Read the model definition and answer for the solid it produces. Units are mm, in the model's axes. A direction names the side the tool comes from. Coordinates: 2 decimals unless noted, no trailing zeros. Loops run counter-clockwise (first coordinate to the right, second up) from the corner with the lowest first, then second, coordinate; pieces in that order, holes last. Notation, with made-up numbers: M 48,38 L 98,38 A14 cw 98,48 Z; hole C 71.5,60 d11. An arc over 180 degrees is marked long. Put each result on its own line as item: value.
from build123d import *

# Parameters (mm, degrees)
BOSS_SWITCH_BODY_DEPTH            = 3
SKETCH1_W                         = 2.994375291
SKETCH1_H                         = 2.409101515
SKETCH1_W_2                       = 3.994375291
SKETCH1_H_2                       = 3.957767538
BOSS_FLANGE_WIDTH_DEPTH           = 5
BOSS_FLANGE_HEIGHT_REACH          = 36.354
SKETCH2_W                         = 4
SKETCH2_H                         = 3.957767538
SKETCH2_W_2                       = 8
SKETCH2_H_2                       = 1.451333978
SKETCH17_W                        = 15.1675
SKETCH17_H                        = 4
BOSS_FLANGE_SUPPORT_DEPTH         = 13.053634428
CUT_WALL_GAP_DEPTH                = 1
TAP_DRILL_FOR_M2X0_4_TAP1_D       = 1.6
M2_CLEARANCE_HOLE2_D              = 2.4
M2_CLEARANCE_HOLE2_DEPTH          = 13.462735941
CHAMFER_FLANGE_SUPPORT_3_SIZE     = 1
FILLET1_R                         = 1
FILLET2_R                         = 0.5
SKETCH28_W                        = 5.9675
SKETCH28_H                        = 12.095866891
CUT_PRINT_SUPPORT_CLEARANCE_DEPTH = 33.624103931


with BuildPart() as part:
    # Sketch-SwitchBossUp → Boss-Switch Body (new body)
    with BuildSketch(Plane.XY):
        with BuildLine():
            Line((-5.697895702, 26.949658376), (-5.524247524, 25.964850623))
            ThreePointArc((-5.524247524, 25.964850623), (-6.169751391, 25.553619307), (-6.3354071, 24.806394693))
            Line((-6.3354071, 24.806394693), (-4.07798079, 12.003893904))
            ThreePointArc((-4.07798079, 12.003893904), (-3.666749473, 11.358390037), (-2.919524859, 11.192734328))
            Line((-2.919524859, 11.192734328), (-2.816117912, 10.606284387))
            Line((-2.816117912, 10.606284387), (-1.811990528, 10.217060362))
            Line((-1.811990528, 10.217060362), (-1.182618868, 9.973100706))
            Line((-1.182618868, 9.973100706), (-1.735258621, 8.547390389))
            ThreePointArc((-1.735258621, 8.547390389), (-1.752158006, 8.457034961), (-1.735258621, 8.366679532))
            Line((-1.735258621, 8.366679532), (-1.182618868, 6.940969215))
            Line((-1.182618868, 6.940969215), (-1.811990528, 6.697009559))
            Line((-1.811990528, 6.697009559), (-0.547014535, 3.433600952))
            Line((-0.547014535, 3.433600952), (0.082357125, 3.677560608))
            Line((0.082357125, 3.677560608), (0.805200549, 1.81275569))
            Line((0.805200549, 1.81275569), (-0.12720191, 1.451333978))
            Line((-0.12720191, 1.451333978), (-0.12720191, 0))
            Line((-0.12720191, 0), (2.867173381, 0))
            Line((2.867173381, 0), (2.867173381, 2.409101515))
            Line((2.867173381, 2.409101515), (2.343664607, 2.409101515))
            Line((2.343664607, 2.409101515), (1.411262148, 2.047679803))
            Line((1.411262148, 2.047679803), (0.688418723, 3.912484721))
            Line((0.688418723, 3.912484721), (1.317790383, 4.156444377))
            Line((1.317790383, 4.156444377), (1.13533703, 4.627140933))
            Line((1.13533703, 4.627140933), (3.197473995, 5.426475025))
            Line((3.197473995, 5.426475025), (3.197473995, 6.761927069))
            Line((3.197473995, 6.761927069), (2.297289747, 7.748445958))
            Line((2.297289747, 7.748445958), (0.235267743, 6.949156428))
            Line((0.235267743, 6.949156428), (0.05281439, 7.419852984))
            Line((0.05281439, 7.419852984), (-0.57655727, 7.175893328))
            Line((-0.57655727, 7.175893328), (-1.038134762, 8.366679532))
            ThreePointArc((-1.038134762, 8.366679532), (-1.055034148, 8.457034961), (-1.038134762, 8.547390389))
            Line((-1.038134762, 8.547390389), (-0.57655727, 9.738176593))
            Line((-0.57655727, 9.738176593), (0.05281439, 9.494216937))
            Line((0.05281439, 9.494216937), (1.317790383, 12.757625544))
            Line((1.317790383, 12.757625544), (0.688418723, 13.0015852))
            Line((0.688418723, 13.0015852), (1.411262148, 14.866390118))
            Line((1.411262148, 14.866390118), (2.343664607, 14.504968406))
            Line((2.343664607, 14.504968406), (2.867173381, 14.504968406))
            Line((2.867173381, 14.504968406), (2.867173381, 18.462735944))
            Line((2.867173381, 18.462735944), (-0.111637615, 18.462735944))
            Line((-0.111637615, 18.462735944), (-1.12720191, 18.462735944))
            Line((-1.12720191, 18.462735944), (-1.12720191, 15.462735944))
            Line((-1.12720191, 15.462735944), (-0.12720191, 15.462735944))
            Line((-0.12720191, 15.462735944), (0.805200549, 15.101314231))
            Line((0.805200549, 15.101314231), (0.082357125, 13.236509313))
            Line((0.082357125, 13.236509313), (-0.547014535, 13.480468969))
            Line((-0.547014535, 13.480468969), (-1.059112089, 12.159350171))
            Line((-1.059112089, 12.159350171), (-2.346896051, 19.462735944))
            Line((-2.346896051, 19.462735944), (3.767173381, 19.462735944))
            Line((3.767173381, 19.462735944), (3.767173381, 25.857619356))
            Line((3.767173381, 25.857619356), (1.767173381, 25.857619356))
            Line((1.767173381, 25.857619356), (1.767173381, 21.462735944))
            Line((1.767173381, 21.462735944), (-2.699550012, 21.462735944))
            Line((-2.699550012, 21.462735944), (-3.728280196, 27.296954732))
            ThreePointArc((-3.728280196, 27.296954732), (-2.874356585, 27.992742953), (-2.319025652, 28.944012807))
            ThreePointArc((-2.319025652, 28.944012807), (-2.76728001, 29.905297381), (-3.728564583, 29.457043022))
            ThreePointArc((-3.728564583, 29.457043022), (-4.944660137, 28.436617692), (-6.436422172, 28.97957467))
            ThreePointArc((-6.436422172, 28.97957467), (-7.493046212, 29.072017295), (-7.585488837, 28.015393255))
            ThreePointArc((-7.585488837, 28.015393255), (-6.738295005, 27.311426358), (-5.697895702, 26.949658376))
        make_face()
    extrude(amount=BOSS_SWITCH_BODY_DEPTH)

    # Sketch1 → Boss-Flange Width (add)
    with BuildSketch(Plane(origin=(0, 0, 0), x_dir=(-1, 0, 0), z_dir=(0, 0, -1))):
        with Locations((-1.369985736, 1.204550758)):
            Rectangle(SKETCH1_W, SKETCH1_H)
        with Locations((-0.869985736, 16.483852175)):
            Rectangle(SKETCH1_W_2, SKETCH1_H_2)
    extrude(amount=BOSS_FLANGE_WIDTH_DEPTH)

    # Boss-Flange Height: up to this face of the body (flat: up to its plane)
    boss_flange_height_end = Plane(part.part.faces().sort_by_distance((-0.12720191, 1.077409098, -1.438016547))[0])
    # Sketch2 → Boss-Flange Height (add, up to the picked face)
    with BuildSketch(Plane(origin=(-12.300326619, 0, 0), x_dir=(0, 0, -1), z_dir=(1, 0, 0)), mode=Mode.PRIVATE) as boss_flange_height_sk1:
        with Locations((3, 16.483852175)):
            Rectangle(SKETCH2_W, SKETCH2_H)
    boss_flange_height_tool1 = split(extrude(boss_flange_height_sk1.sketch, amount=BOSS_FLANGE_HEIGHT_REACH, mode=Mode.PRIVATE), bisect_by=boss_flange_height_end, keep=Keep.BOTH, mode=Mode.PRIVATE)
    # Sketch2 → Boss-Flange Height (add, up to the picked face)
    with BuildSketch(Plane(origin=(-12.300326619, 0, 0), x_dir=(0, 0, -1), z_dir=(1, 0, 0)), mode=Mode.PRIVATE) as boss_flange_height_sk2:
        with Locations((1, 0.725666989)):
            Rectangle(SKETCH2_W_2, SKETCH2_H_2)
    boss_flange_height_tool2 = split(extrude(boss_flange_height_sk2.sketch, amount=BOSS_FLANGE_HEIGHT_REACH, mode=Mode.PRIVATE), bisect_by=boss_flange_height_end, keep=Keep.BOTH, mode=Mode.PRIVATE)
    add(boss_flange_height_tool1.solids().sort_by(Axis((-12.300327, 16.483852, -3), (1, 0, 0)))[0])
    add(boss_flange_height_tool2.solids().sort_by(Axis((-12.300327, 0.725667, -1), (1, 0, 0)))[0])

    # Sketch17 → Boss-Flange Support (add)
    with BuildSketch(Plane.XZ.offset(-1.451333978)):
        with Locations((-4.716576619, -3)):
            Rectangle(SKETCH17_W, SKETCH17_H)
    extrude(amount=-BOSS_FLANGE_SUPPORT_DEPTH)

    # Sketch27 → Cut-Wall Gap (cut)
    with BuildSketch(Plane.XY):
        Polygon((-0.12720191, 15.462735944), (2.343664607, 14.504968406), (-1.12720191, 14.504968406), (-1.12720191, 15.462735944), align=None)
        Polygon((2.343664607, 2.409101515), (-0.12720191, 2.409101515), (-0.12720191, 1.451333978), align=None)
    extrude(amount=-CUT_WALL_GAP_DEPTH, mode=Mode.SUBTRACT)

    # Tap Drill for M2x0.4 Tap1 (through all)
    with Locations(Plane(origin=(0, 0, 0), x_dir=(-1, 0, 0), z_dir=(0, -1, 0))):
        with Locations((9.300326619, 3), (5.300326619, 3)):
            Hole(TAP_DRILL_FOR_M2X0_4_TAP1_D / 2)

    # M2 Clearance Hole2
    with Locations(Plane.XZ):
        with Locations((-9.300326619, -3), (-5.300326619, -3)):
            Hole(M2_CLEARANCE_HOLE2_D / 2, depth=M2_CLEARANCE_HOLE2_DEPTH)

    # Chamfer-Flange Support 3
    chamfer_flange_support_3_edges = [part.edges().sort_by_distance(p)[0] for p in [
        (-6.213764264, 1.451333978, -1),
    ]]
    chamfer(chamfer_flange_support_3_edges, length=CHAMFER_FLANGE_SUPPORT_3_SIZE)

    # Fillet1
    fillet1_edges = [part.edges().sort_by_distance(p)[0] for p in [
        (-2.816117912, 10.606284387, 1.5),
    ]]
    fillet(fillet1_edges, radius=FILLET1_R)

    # Fillet2
    fillet2_edges = [part.edges().sort_by_distance(p)[0] for p in [
        (-1.811990528, 6.697009559, 1.5),
    ]]
    fillet(fillet2_edges, radius=FILLET2_R)

    # Sketch28 → Cut-Print Support Clearance (cut, through all)
    with BuildSketch(Plane.XY.offset(-1)):
        with Locations((-0.116576619, 8.457034961)):
            Rectangle(SKETCH28_W, SKETCH28_H)
    extrude(amount=-CUT_PRINT_SUPPORT_CLEARANCE_DEPTH, mode=Mode.SUBTRACT)


solid = part.part
1) Straight lines are drawn through the part: line 1 (X direction, y = 16.95, z = -3); line 2 (Y direction, x = 1.25, z = -1.25); line 3 (Z direction, x = -3.25, y = 11.75). For each, find the intervals that lie inside material, in ascending order. Write a range as [from, to].
Answer list:
line 1: x = [-12.3, -10.1], [-8.5, -6.1], [-4.5, 2.87]
line 2: y = [0, 2.41], [14.5, 18.46]
line 3: z = [-5, -1], [0, 3]
2) Given pin 1 Ø1.9 at (x, z) = (-10, -2.5) entering from -Y; pin 2 Ø3 at (x, z) = (-7, -3.5) entering from +Y; pin 3 Ø2.5 at (y, z) = (17, 2) entering from -X; pin 4 Ø1.6 at (x, z) = (3, 2) entering from +Y, each flat-ended and moving along its own axis, determine where each tip first touches the part or whether it passes through.
Answer list:
pin 1: stops at y = 0
pin 2: stops at y = 18.46
pin 3: stops at x = -5.18
pin 4: stops at y = 25.86
3) Determine the mould class of faces 6 (the cylindrical face through (-6.163, 25.563, 1.479)), 7 (the flat face through (-0.8, 12.83, 1.48)), 8 (the flat face through (3.197, 6, 1)), 9 (the flat face through (-5, 0, -1)) for opening direction X: released by +X, released by -X, zero draft, split by the parting line, or undercut.
Answer list:
face 6: released by -X
face 7: undercut
face 8: released by +X
face 9: zero draft
4) Find section B-B, the plane y = 16.25. Write down the section's boundary in (x, z), plus the area to 3 significant figures.
Answer list:
outline: M -12.3,-5 L 2.87,-5 L 2.87,3 L -1.13,3 L -1.13,-1 L -12.3,-1 Z; M -4.83,0 L -1.78,0 L -1.78,3 L -4.83,3 Z; hole C -9.3,-3 d1.6; hole C -5.3,-3 d1.6
area: 81.8 mm^2
5) Which of the six approach directions +Z, -Z, +X, -X, +Y, -Y give full straight-line access (tool end or side, diameter ignored) to faces 1 (the flat face through (0.45, 14.18, 1.48)), 2 (the flat face through (2.15, 5.02, 1.48)), 3 (the flat face through (-2.5, 17, 0)), 4 (the flat face through (0, 14.505, -3)), 5 (the flat face through (-0.811, 9.134, 1.479))?
Answer list:
face 1: +Z
face 2: +Z, -Z, +X
face 3: -X
face 4: -Z, +X
face 5: +Z, -Z
6) Find section A-A, the plane z = -3. Write down the section's boundary in (x, y).
Answer list:
outline: M -12.3,0 L -10.5,0 L -10.5,13.46 L -10.1,13.46 L -10.1,18.46 L -12.3,18.46 Z; M -8.5,13.46 L -8.1,13.46 L -8.1,0 L -6.5,0 L -6.5,13.46 L -6.1,13.46 L -6.1,18.46 L -8.5,18.46 Z; M -4.5,13.46 L -4.1,13.46 L -4.1,0 L 2.87,0 L 2.87,2.41 L -3.1,2.41 L -3.1,14.5 L 2.87,14.5 L 2.87,18.46 L -4.5,18.46 Z
